The model under review builds one solid part; all positions refer to its coordinate system, in mm. A direction names the side the tool comes from. Round coordinates to 2 decimals unless told otherwise and drop trailing zeros. Loops run counter-clockwise (first coordinate to the right, second up) from the corner with the lowest first, then second, coordinate; pieces in that order, holes last. Notation, with made-up numbers: (13, 46.25) -> (67, 46.25) arc R11 ccw to (67, 52.25) -> close; hole circle Ø7 at (28, 87). An arc over 180 degrees is marked (long way). Return JSON: item names as keys, results as strings. Group by question number.
```python
from build123d import *

# Parameters (mm, degrees)
SKETCH_1_R          = 63
SKETCH_1_R_2        = 1.25
EXTRUDE_1_DEPTH     = 5
SKETCH_2_R          = 12
CUT_EXTRUDE_4_DEPTH = 5
SKETCH_3_R          = 9.5
CUT_EXTRUDE_5_DEPTH = 10
SKETCH_4_R          = 11
CUT_EXTRUDE_6_DEPTH = 1


with BuildPart() as part:
    # 草图1 → 凸台-拉伸1 (new body)
    with BuildSketch(Plane.XY):
        Circle(SKETCH_1_R)
        with Locations((0, 55)):
            Circle(SKETCH_1_R_2, mode=Mode.SUBTRACT)
        with Locations((47.631397208, 27.5)):
            Circle(SKETCH_1_R_2, mode=Mode.SUBTRACT)
        with Locations((47.631397208, -27.5)):
            Circle(SKETCH_1_R_2, mode=Mode.SUBTRACT)
        with Locations((0, -55)):
            Circle(SKETCH_1_R_2, mode=Mode.SUBTRACT)
        with Locations((-47.631397208, -27.5)):
            Circle(SKETCH_1_R_2, mode=Mode.SUBTRACT)
        with Locations((-47.631397208, 27.5)):
            Circle(SKETCH_1_R_2, mode=Mode.SUBTRACT)
        with Locations((-42.132444372, 35.353318533)):
            Circle(SKETCH_1_R_2, mode=Mode.SUBTRACT)
        with Locations((9.550649772, 54.164426416)):
            Circle(SKETCH_1_R_2, mode=Mode.SUBTRACT)
        with Locations((51.683094143, 18.811107883)):
            Circle(SKETCH_1_R_2, mode=Mode.SUBTRACT)
        with Locations((42.132444372, -35.353318533)):
            Circle(SKETCH_1_R_2, mode=Mode.SUBTRACT)
        with Locations((-9.550649772, -54.164426416)):
            Circle(SKETCH_1_R_2, mode=Mode.SUBTRACT)
        with Locations((-51.683094143, -18.811107883)):
            Circle(SKETCH_1_R_2, mode=Mode.SUBTRACT)
    extrude(amount=EXTRUDE_1_DEPTH)

    # 草图2 → 切除-拉伸4 (cut)
    with BuildSketch(Plane.XY.offset(5)):
        with Locations((39.073033019, 0)):
            Circle(SKETCH_2_R)
    extrude(amount=-CUT_EXTRUDE_4_DEPTH, mode=Mode.SUBTRACT)

    # 草图3 → 切除-拉伸5 (cut)
    with BuildSketch(Plane.XY.offset(5)):
        Circle(SKETCH_3_R)
    extrude(amount=-CUT_EXTRUDE_5_DEPTH, mode=Mode.SUBTRACT)

    # 草图4 → 切除-拉伸6 (cut)
    with BuildSketch(Plane.XY.offset(5)):
        Circle(SKETCH_4_R)
    extrude(amount=-CUT_EXTRUDE_6_DEPTH, mode=Mode.SUBTRACT)


solid = part.part
```
1. We need section B-B, the plane x = 29.5. Write out the cut boundary in (y, z), then the cut area to 3 significant figures.
2. We need section C-C, the plane z = 3.2. Give the number of separate pieces and of enclosed holes in the cut face, then the cut area to 3 significant figures.
3. For P1, Ø2, axis at x = 0, y = -55, coming from the -Z side; P2, Ø3, axis at y = -34.5, z = 3.5, coming from the +X side; P3, Ø1, axis at y = -30, z = 0.5, coming from the +X side, all flat-tipped, find the tip position at first contact; note any pin that passes through.
4. Tool access review of faces 4 (the face through (-2.38, -10.74, 4.51)), 5 (the face through (50.52, 3.6, 2.54)): name each direction out of +Z, -Z, +X, -X, +Y, -Y from which nothing blocks a thin tool from reaching the whole face with its end or side.
5. Wall thickness on line 1 (Y direction, x = 0, z = 1.2); line 2 (Y direction, x = 0, z = 4.5); line 3 (X direction, y = -34.5, z = 2): over which ranges is each line inside the solid? List them lowest first.
6. We need section D-D, the plane x = -4.5. Write out the cut boundary in (y, z).
7. Draft analysis for pull direction X (two halves, no side actions). For faces 1 (the face through (-1, -13, 5)), 2 (the face through (4.38, -8.43, 2.03)), 3 (the face through (-8.201, 62.464, 2.465)), state which applies: pulls with the +X half, pulls with the -X half, needs draft (parallel to the pull), parting line crosses it, or undercut.
8. We need section A-A, the plane y = 0. Write out the cut boundary in (x, z), then the cut area to 3 significant figures.
Check sheet entries:
{
 "1": {"outline": "(-55.67, 0) -> (-7.24, 0) -> (-7.24, 5) -> (-55.67, 5) -> close; (7.24, 0) -> (55.67, 0) -> (55.67, 5) -> (7.24, 5) -> close", "area": "484 mm²"},
 "2": {"separate pieces": "1", "enclosed holes": "14", "area": "11,700 mm²"},
 "3": {"P1": "passes through", "P2": "stops at x = 53.67", "P3": "stops at x = 55.67"},
 "4": {"face 4": "+Z", "face 5": "+Z, -Z"},
 "5": {"line 1": "y = -63 to -56.25, -53.75 to -9.5, 9.5 to 53.75, 56.25 to 63", "line 2": "y = -63 to -56.25, -53.75 to -11, 11 to 53.75, 56.25 to 63", "line 3": "x = -52.71 to 41.22, 43.05 to 52.71"},
 "6": {"outline": "(-62.84, 0) -> (-8.37, 0) -> (-8.37, 4) -> (-10.04, 4) -> (-10.04, 5) -> (-62.84, 5) -> close; (8.37, 0) -> (62.84, 0) -> (62.84, 5) -> (10.04, 5) -> (10.04, 4) -> (8.37, 4) -> close"},
 "7": {"face 1": "needs draft", "face 2": "undercut", "face 3": "parting line crosses it"},
 "8": {"outline": "(-63, 0) -> (-9.5, 0) -> (-9.5, 4) -> (-11, 4) -> (-11, 5) -> (-63, 5) -> close; (9.5, 0) -> (27.07, 0) -> (27.07, 5) -> (11, 5) -> (11, 4) -> (9.5, 4) -> close; (51.07, 0) -> (63, 0) -> (63, 5) -> (51.07, 5) -> close", "area": "412 mm²"}
}
